```python
from build123d import *

# Parameters (mm, degrees)
BOSS_EXTRUDE1_DEPTH      = 57.15
BOSS_EXTRUDE1_DEPTH_BACK = 44.45
SKETCH3_R                = 3.556
CUT_EXTRUDE1_DEPTH       = 13.7


with BuildPart() as part:
    # Sketch1 → Boss-Extrude1 (new body, two sides)
    with BuildSketch(Plane(origin=(0, 0, 0), x_dir=(0, 0, -1), z_dir=(1, 0, 0))) as boss_extrude1_sk:
        Polygon((0, 0), (0, 12.7), (-12.7, 12.7), (-12.7, 11.1125), (-1.5875, 11.1125), (-1.5875, 0), align=None)
    extrude(amount=BOSS_EXTRUDE1_DEPTH)
    extrude(boss_extrude1_sk.sketch, amount=-BOSS_EXTRUDE1_DEPTH_BACK)

    # Sketch3 → Cut-Extrude1 (cut, through all)
    with BuildSketch(Plane(origin=(0, 0, 0), x_dir=(-1, 0, 0), z_dir=(0, 0, -1))):
        with Locations((25.4, 5.08)):
            Circle(SKETCH3_R)
        with Locations((-50.8, 5.08)):
            Circle(SKETCH3_R)
    extrude(amount=-CUT_EXTRUDE1_DEPTH, mode=Mode.SUBTRACT)


solid = part.part
```
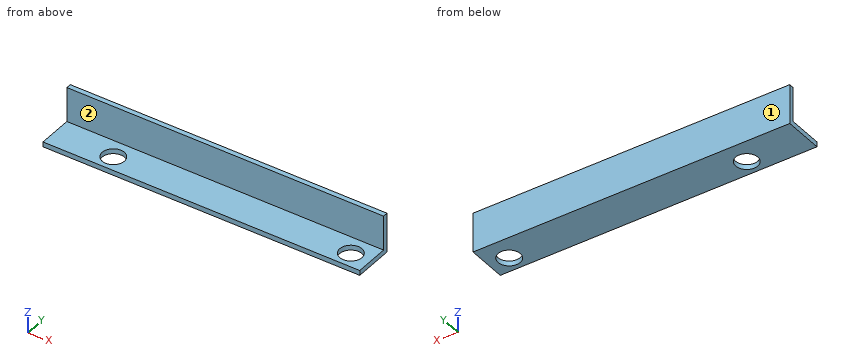
For this review, take the finished solid that the model builds, in its own axes (mm). Face numbers are marked on the shaded views. A direction names the side the tool comes from. Coordinates: 2 decimals unless noted, no trailing zeros. Write each loop counter-clockwise with the first axis right and the second up, starting at its lowest first coordinate (ties: lowest second). Pieces come first, ordered by that corner, then holes. Notation, with made-up numbers: (6, -4) - (56, -4) arc R28 ccw to (56, 31) - close; hole circle Ø8 at (-14.75, 15.25). An arc over 180 degrees is marked (long way). Answer in a Markdown table with one row per item. Add a question column.
Q1. We need section D-D, the plane x = 5. State the section outline as (y, z) points.
Q2. Tool access review of the marked faces 1 and 2: name each direction out of +Z, -Z, +X, -X, +Y, -Y from which nothing blocks a thin tool from reaching the whole face with its end or side.
Q3. We need section B-B, the plane x = -25.4. State the section outline as (y, z) points, and give its area (3 significant figures).
Q4. We need section C-C, the plane z = 8. State the section outline as (x, y) points, and give its area (3 significant figures).
Q5. For probe 1 along X at (y, z) = (8.25, 1); probe 2 along Y at (x, z) = (-25.4, 0.4); probe 3 along Z at (x, y) = (42, 3.5), list the stretches that pass through material, from the lowest coordinate up.
Q6. We need section A-A, the plane y = 5.08. State the section outline as (x, z) points, and give its area (3 significant figures).
Q7. For P1, Ø2, axis at x = 36.5, z = 10, coming from the -Y side; P2, Ø4.5, axis at x = -25.4, y = 5.08, coming from the +Z side, all flat-tipped, find the tip position at first contact; note any pin that passes through.
Answer list:
| question | item | result |
|---|---|---|
| 1 | outline | (0, 0) - (12.7, 0) - (12.7, 12.7) - (11.11, 12.7) - (11.11, 1.59) - (0, 1.59) - close |
| 2 | face 1 | +Z, -Z, +X, -X, +Y |
| 2 | face 2 | +Z, +X, -X, -Y |
| 3 | outline | (0, 0) - (1.52, 0) - (1.52, 1.59) - (0, 1.59) - close; (8.64, 0) - (12.7, 0) - (12.7, 12.7) - (11.11, 12.7) - (11.11, 1.59) - (8.64, 1.59) - close |
| 3 | area | 26.5 mm2 |
| 4 | outline | (-44.45, 11.11) - (57.15, 11.11) - (57.15, 12.7) - (-44.45, 12.7) - close |
| 4 | area | 161 mm2 |
| 5 | probe 1 | x = -44.45 to -27.01, -23.79 to 49.19, 52.41 to 57.15 |
| 5 | probe 2 | y = 0 to 1.52, 8.64 to 12.7 |
| 5 | probe 3 | z = 0 to 1.59 |
| 6 | outline | (-44.45, 0) - (-28.96, 0) - (-28.96, 1.59) - (-44.45, 1.59) - close; (-21.84, 0) - (47.24, 0) - (47.24, 1.59) - (-21.84, 1.59) - close; (54.36, 0) - (57.15, 0) - (57.15, 1.59) - (54.36, 1.59) - close |
| 6 | area | 139 mm2 |
| 7 | P1 | stops at y = 11.11 |
| 7 | P2 | passes through |
